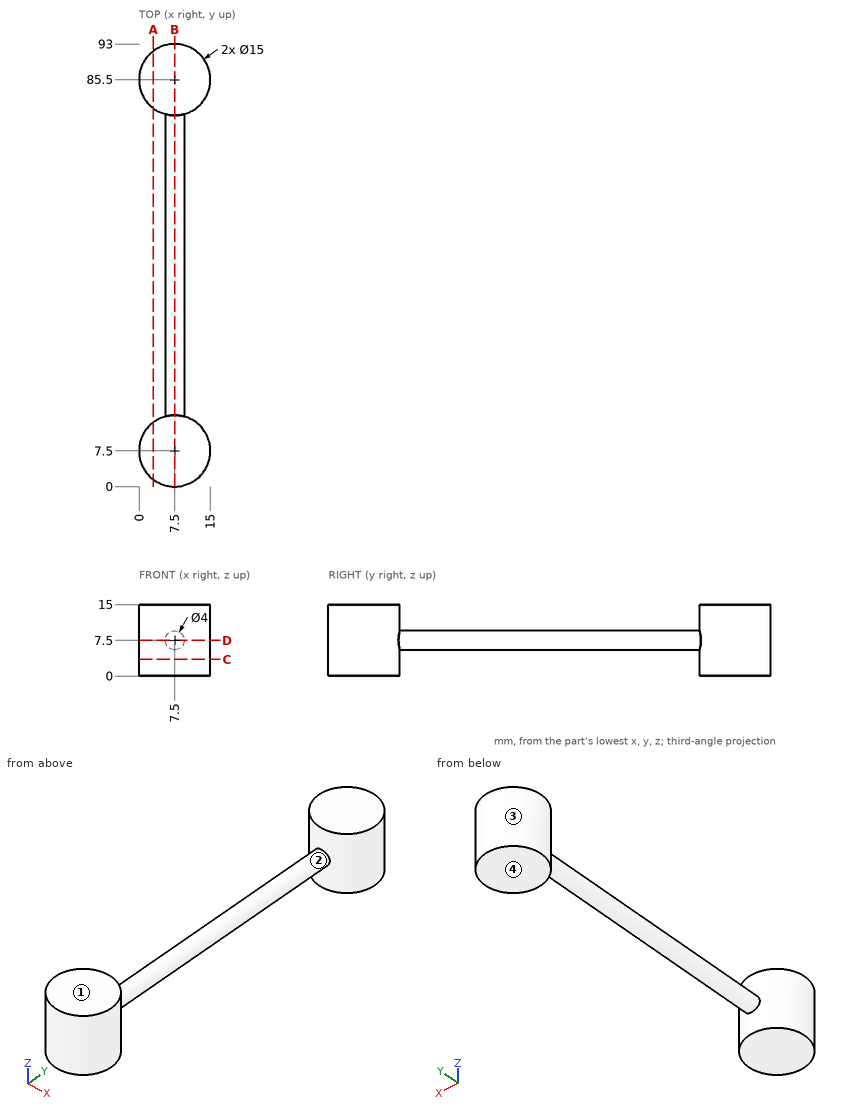
The drawing under review shows one solid part. Ordinate dimensions are in mm from its lowest x, y, z. A direction names the side the tool comes from. Give positions to 0.01 mm unless a question says otherwise; leave off trailing zeros. Order: outer loops, then holes, each group sorted by start corner. A loop starts at its lowest first (then second) coordinate and runs counter-clockwise, first axis right, second up. Notation, with made-up numbers: M 39.25,53 L 56.25,53 A19 ccw 56.25,72 Z; hole C 79,80 d7. An arc over 180 degrees is marked long. One line per question, with ' | ' between items. Start each with the question number.
Q1. We need section A-A (x = 3). Write out the cut boundary in (y, z).
Q2. For pin 1 Ø3 at (x, y) = (5, 52.5) entering from +Z; pin 2 Ø4 at (x, z) = (4, 4.5) entering from +Y; pin 3 Ø4 at (y, z) = (58.5, 4.5) entering from -X, all flat-tipped, find the tip position at first contact; note any pin that passes through.
Q3. For L1, parallel to Y at x = 5.25, z = 1; L2, parallel to Y at x = 9.25, z = 5; L3, parallel to X at y = 59.5, z = 7.5, list the stretches that pass through material, from the lowest coordinate up. Write a range as [from, to].
Q4. Machinability: for the marked faces 1 and 2, which of the approach directions +Z, -Z, +X, -X, +Y, -Y give a long, thin tool a straight path to every point of the face, cutting with its end or side? Answer none if there is none.
Q5. The part is to be moulded in two halves that separate along Y. For the marked faces 3 and 4, say which applies: +Y half, -Y half, draft (parallel to the pull), parting line (faces both ways), or undercut.
Q6. We need section C-C (z = 3.5). Write out the cut boundary in (x, y).
Q7. We need section B-B (x = 7.5). Write out the cut boundary in (y, z).
Q8. We need section D-D (z = 7.5). Write out the cut boundary in (x, y).
Returned:
1) outline: M 1.5,0 L 13.5,0 L 13.5,15 L 1.5,15 Z; M 79.5,0 L 91.5,0 L 91.5,15 L 79.5,15 Z
2) pin 1: z = 9.23 | pin 2: y = 92.85 | pin 3: x = 5.77
3) L1: [0.35, 14.65], [78.35, 92.65] | L2: [0.21, 14.79], [78.21, 92.79] | L3: [5.5, 9.5]
4) face 1: +Z, +X, -X, +Y, -Y | face 2: none
5) face 3: undercut | face 4: draft
6) outline: C 7.5,7.5 d15; C 7.5,85.5 d15
7) outline: M 0,0 L 15,0 L 15,5.5 L 78,5.5 L 78,0 L 93,0 L 93,15 L 78,15 L 78,9.5 L 15,9.5 L 15,15 L 0,15 Z
8) outline: M 5.5,14.73 A7.5 ccw long 9.5,14.73 L 9.5,78.27 A7.5 ccw long 5.5,78.27 Z
